For this review, take the finished solid that the model builds, in its own axes (mm). A direction names the side the tool comes from. Coordinates: 2 decimals unless noted, no trailing zeros. Loops run counter-clockwise (first coordinate to the right, second up) from the corner with the lowest first, then second, coordinate; pieces in that order, holes last. Notation, with made-up numbers: (67.25, 13.25) -> (89.25, 13.25) arc R15 ccw to (89.25, 37.25) -> close; hole circle Ø5 at (-25.5, 40.25). An arc over 180 degrees is marked (long way). Answer in a Markdown table with one row per item.
from build123d import *

# Parameters (mm, degrees)
SKETCH_1_R      = 42
SKETCH_1_R_2    = 25
SKETCH_1_R_3    = 3.25
EXTRUDE_1_DEPTH = 6
EXTRUDE_START   = -3
SKETCH_2_R      = 62.5
SKETCH_2_R_2    = 42
EXTRUDE_2_DEPTH = 20


with BuildPart() as part:
    # 草图1 → 凸台-拉伸1 (new body)
    with BuildSketch(Plane.XY):
        Circle(SKETCH_1_R)
        Circle(SKETCH_1_R_2, mode=Mode.SUBTRACT)
        with Locations((0, 35)):
            Circle(SKETCH_1_R_3, mode=Mode.SUBTRACT)
        with Locations((30.310889132, 17.5)):
            Circle(SKETCH_1_R_3, mode=Mode.SUBTRACT)
        with Locations((30.310889132, -17.5)):
            Circle(SKETCH_1_R_3, mode=Mode.SUBTRACT)
        with Locations((0, -35)):
            Circle(SKETCH_1_R_3, mode=Mode.SUBTRACT)
        with Locations((-30.310889132, -17.5)):
            Circle(SKETCH_1_R_3, mode=Mode.SUBTRACT)
        with Locations((-30.310889132, 17.5)):
            Circle(SKETCH_1_R_3, mode=Mode.SUBTRACT)
    extrude(amount=EXTRUDE_1_DEPTH)

    # 草图2 → 凸台-拉伸2 (add, symmetric)
    with BuildSketch(Plane.XY.offset(6).offset(EXTRUDE_START)):
        Circle(SKETCH_2_R)
        Circle(SKETCH_2_R_2, mode=Mode.SUBTRACT)
    extrude(amount=EXTRUDE_2_DEPTH, both=True)


solid = part.part
Item 1: For L1, parallel to Y at x = 0, z = 3.8; L2, parallel to X at y = 17, z = 2; L3, parallel to X at y = 16, z = 1, list the stretches that pass through material, from the lowest coordinate up.
Worked answers:
| item | result |
|---|---|
| L1 | -62.5 to -38.25, -31.75 to -25, 25 to 31.75, 38.25 to 62.5 |
| L2 | -60.14 to -33.52, -27.1 to -18.33, 18.33 to 27.1, 33.52 to 60.14 |
| L3 | -60.42 to -33.19, -27.43 to -19.21, 19.21 to 27.43, 33.19 to 60.42 |
Item 2: For faces 4 (the cylindrical face through (40.06, 12.62, 14.38)), 5 (the cylindrical face through (40.06, 12.62, -8.62)), 6 (the cylindrical face through (32.06, -14.76, 2.96)), list the 3-axis set-ups (+Z, -Z, +X, -X, +Y, -Y) from which the entire face can be reached by the end or side of a thin tool; tool diameter is ignored.
Worked answers:
| item | result |
|---|---|
| face 4 | +Z |
| face 5 | -Z |
| face 6 | +Z, -Z |
Item 3: Insertion check: pin 1 (2 mm diameter, centred on y = -23.5, z = 0.5, fed in from -X); pin 2 (8.5 mm diameter, centred on x = 30.31, y = 17.5, fed in from -Z); pin 3 (10.5 mm diameter, centred on x = -30.31, y = -17.5, fed in from +Z). Each pin has a flat end and moves straight along its axis. Give the tip position at first contact, or say it passes through.
Worked answers:
| item | result |
|---|---|
| pin 1 | x = -58.31 |
| pin 2 | z = 0 |
| pin 3 | z = 6 |
Item 4: Take a section at C-C, the plane x = -22. State the section outline as (y, z) points.
Worked answers:
| item | result |
|---|---|
| outline | (-58.5, -17) -> (-35.78, -17) -> (-35.78, 0) -> (-11.87, 0) -> (-11.87, 6) -> (-35.78, 6) -> (-35.78, 23) -> (-58.5, 23) -> close; (11.87, 0) -> (35.78, 0) -> (35.78, -17) -> (58.5, -17) -> (58.5, 23) -> (35.78, 23) -> (35.78, 6) -> (11.87, 6) -> close |
Item 5: Take a section at B-B, the plane y = 7. State the section outline as (x, z) points.
Worked answers:
| item | result |
|---|---|
| outline | (-62.11, -17) -> (-41.41, -17) -> (-41.41, 0) -> (-24, 0) -> (-24, 6) -> (-41.41, 6) -> (-41.41, 23) -> (-62.11, 23) -> close; (24, 0) -> (41.41, 0) -> (41.41, -17) -> (62.11, -17) -> (62.11, 23) -> (41.41, 23) -> (41.41, 6) -> (24, 6) -> close |
Item 6: The part is to be moulded in two halves that separate along Y. For faces 1 (the cylindrical face through (-62.44, 2.75, 3.28)), 2 (the flat face through (18, -18, 6)), 3 (the flat face through (41, -13, 23)), say which applies: +Y half, -Y half, draft (parallel to the pull), parting line (faces both ways), or undercut.
Worked answers:
| item | result |
|---|---|
| face 1 | parting line |
| face 2 | undercut |
| face 3 | draft |
Item 7: Take a section at A-A, the plane x = 0. State the section outline as (y, z) points, and give its area (3 significant figures).
Worked answers:
| item | result |
|---|---|
| outline | (-62.5, -17) -> (-42, -17) -> (-42, 0) -> (-38.25, 0) -> (-38.25, 6) -> (-42, 6) -> (-42, 23) -> (-62.5, 23) -> close; (-31.75, 0) -> (-25, 0) -> (-25, 6) -> (-31.75, 6) -> close; (25, 0) -> (31.75, 0) -> (31.75, 6) -> (25, 6) -> close; (38.25, 0) -> (42, 0) -> (42, -17) -> (62.5, -17) -> (62.5, 23) -> (42, 23) -> (42, 6) -> (38.25, 6) -> close |
| area | 1,770 mm² |
Item 8: Take a section at D-D, the plane z = 12. State the section outline as (x, y) points, and give its area (3 significant figures).
Worked answers:
| item | result |
|---|---|
| outline | circle Ø125 at (0, 0); hole circle Ø84 at (0, 0) |
| area | 6,730 mm² |
